```python
from build123d import *

# Parameters (mm, degrees)
SKETCH1_R           = 45.85
BOSS_EXTRUDE1_DEPTH = 5
SKETCH2_R           = 1.565
CUT_EXTRUDE1_DEPTH  = 10
SKETCH3_R           = 1.5
SKETCH3_R_2         = 7
CUT_EXTRUDE2_DEPTH  = 10
BOSS_EXTRUDE2_START = -5
BOSS_EXTRUDE2_DEPTH = 5
SKETCH5_W           = 150
SKETCH5_H           = 8
BOSS_EXTRUDE3_DEPTH = 75
FILLET1_R           = 3
FILLET2_R           = 3


with BuildPart() as part:
    # Sketch1 → Boss-Extrude1 (new body)
    with BuildSketch(Plane(origin=(0, 0, 0), x_dir=(1, 0, 0), z_dir=(0, 1, 0))):
        with Locations(Location((0, 0, 0), (0, 0, 270))):
            Circle(SKETCH1_R)
    extrude(amount=BOSS_EXTRUDE1_DEPTH)

    # Sketch2 → Cut-Extrude1 (cut)
    with BuildSketch(Plane(origin=(0, 5, 0), x_dir=(1, 0, 0), z_dir=(0, 1, 0))):
        with Locations(Location((0, 42.5, 0), (0, 0, 270))):
            Circle(SKETCH2_R)
        with Locations(Location((36.806079661, -21.25, 0), (0, 0, 270))):
            Circle(SKETCH2_R)
        with Locations(Location((-36.806079661, -21.25, 0), (0, 0, 270))):
            Circle(SKETCH2_R)
    extrude(amount=-CUT_EXTRUDE1_DEPTH, mode=Mode.SUBTRACT)

    # Sketch3 → Cut-Extrude2 (cut)
    with BuildSketch(Plane(origin=(0, 5, 0), x_dir=(1, 0, 0), z_dir=(0, 1, 0))):
        with Locations(Location((-15.5, 15.5, 0), (0, 0, 270))):
            Circle(SKETCH3_R)
        with Locations(Location((15.5, 15.5, 0), (0, 0, 270))):
            Circle(SKETCH3_R)
        with Locations(Location((15.5, -15.5, 0), (0, 0, 270))):
            Circle(SKETCH3_R)
        with Locations(Location((-15.5, -15.5, 0), (0, 0, 270))):
            Circle(SKETCH3_R)
        with Locations(Location((0, 0, 0), (0, 0, 270))):
            Circle(SKETCH3_R_2)
    extrude(amount=-CUT_EXTRUDE2_DEPTH, mode=Mode.SUBTRACT)

    # Sketch4 → Boss-Extrude2 (add)
    with BuildSketch(Plane(origin=(0, 5, 0), x_dir=(1, 0, 0), z_dir=(0, 1, 0)).offset(BOSS_EXTRUDE2_START)):
        with BuildLine():
            Line((-45.85, 0), (-45.85, -57.708767277))
            Line((-45.85, -57.708767277), (45.85, -57.708767277))
            Line((45.85, -57.708767277), (45.85, 0))
            ThreePointArc((45.85, 0), (0, -45.85), (-45.85, 0))
        make_face()
    extrude(amount=BOSS_EXTRUDE2_DEPTH)

    # Sketch5 → Boss-Extrude3 (add)
    with BuildSketch(Plane(origin=(0, 0, 0), x_dir=(1, 0, 0), z_dir=(0, 1, 0))):
        with Locations((0, -53.708767277)):
            Rectangle(SKETCH5_W, SKETCH5_H)
    extrude(amount=BOSS_EXTRUDE3_DEPTH)

    # Fillet1
    fillet1_edges = [part.edges().sort_by_distance(p)[0] for p in [
        (-45.85, 2.5, 49.708767277),
        (0, 5, 49.708767277),
        (45.85, 2.5, 49.708767277),
    ]]
    fillet(fillet1_edges, radius=FILLET1_R)

    # Fillet2
    fillet2_edges = [part.edges().sort_by_distance(p)[0] for p in [
        (-75, 0, 53.708767277),
        (75, 0, 53.708767277),
        (-75, 75, 53.708767277),
        (75, 75, 53.708767277),
    ]]
    fillet(fillet2_edges, radius=FILLET2_R)


solid = part.part
```
Could you check a few things on this model? Use its own coordinates, in mm. A direction names the side the tool comes from. Coordinates: 2 decimals unless noted, no trailing zeros. Loops run counter-clockwise (first coordinate to the right, second up) from the corner with the lowest first, then second, coordinate; pieces in that order, holes last. Notation, with made-up numbers: M 20,33.25 L 49,33.25 A19 cw 49,59.25 Z; hole C 88,-4 d4. An arc over 180 degrees is marked long. Put each result on its own line as item: value. Start each with the question number.
(1) I need wall thicknesses on line 1 (X direction, y = 2.7, z = 15.5); line 2 (X direction, y = 2, z = 21); line 3 (Z direction, x = -15, y = 3). Which ranges of each line are inside material? Lowest first, please. Write a range as from..to.
(2) Suppose I cut it at A-A on x = 30. Please give me the cut outline in (y, z), then the cut area to 3 significant figures.
(3) Suppose I cut it at D-D on z = 12. Please give me the cut outline in (x, y), then the cut area to 4 significant figures.
(4) Thinking about a two-plate mould opening in Z: for faces 1 (the face through (-0.68, 5.86, 48.81)), 2 (the face through (15.57, 2.54, -17)), 3 (the face through (-74.14, 74.1, 53.65)), which applies, pulls with the +Z half, pulls with the -Z half, needs draft (parallel to the pull), parting line crosses it, or undercut?
(5) Suppose I cut it at B-B on x = 5. Please give me the cut outline in (y, z), then the cut area to 3 significant figures.
(6) Will these pins go through, and if not, where does the flat tip stop? P1, Ø2, axis at x = 25.5, y = 43.5, coming from the -Z side; P2, Ø5, axis at x = 15.5, z = 15.5, coming from the +Y side; P3, Ø1.5, axis at y = 3, z = 30.5, coming from the -X side.
(7) For faces 4 (the face through (35.28, 2.54, 20.91)), 5 (the face through (-1, 5, 10)), which set-ups out of +Z, -Z, +X, -X, +Y, -Y let a thin tool reach every point of the face, with its end or its side?
(8) Suppose I cut it at C-C on y = 50. Please give me the cut outline in (x, z).
Solutions:
1. line 1: x = -45.85..-17, -14..14, 17..45.85
1. line 2: x = -45.85..-38.35, -35.26..35.26, 38.35..45.85
1. line 3: z = -43.33..-16.91, -14.09..14.09, 16.91..57.71
2. outline: M 0,-34.67 L 5,-34.67 L 5,46.71 A3 cw 8,49.71 L 75,49.71 L 75,57.71 L 0,57.71 Z
2. area: 1,020 mm2
3. outline: M -45.85,0 L 45.85,0 L 45.85,5 L -45.85,5 Z
3. area: 458.5 mm2
4. face 1: pulls with the -Z half
4. face 2: undercut
4. face 3: needs draft
5. outline: M 0,-45.58 L 5,-45.58 L 5,-4.9 L 0,-4.9 Z; M 0,4.9 L 5,4.9 L 5,46.71 A3 cw 8,49.71 L 75,49.71 L 75,57.71 L 0,57.71 Z
5. area: 1,030 mm2
6. P1: stops at z = 49.71
6. P2: stops at y = 5
6. P3: stops at x = -45.85
7. face 4: +Y, -Y
7. face 5: -Z, +X, -X, +Y
8. outline: M -75,49.71 L 75,49.71 L 75,57.71 L -75,57.71 Z
